Check sheet for the modelled part. Datum: model origin and axes. Units: mm. A direction names the side the tool comes from. Give positions to 0.01 mm unless a question says otherwise; leave off trailing zeros. Order: outer loops, then holes, each group sorted by start corner. A loop starts at its lowest first (then second) coordinate and runs counter-clockwise, first axis right, second up. Notation, with made-up numbers: (84.5, 45.25) - (130.5, 45.25) arc R13 cw to (130.5, 69.25) - close; hole circle Ø9 at (-12, -22.75). An arc over 180 degrees is marked (long way). Answer in a Markdown table with one row per item.
from build123d import *

# Parameters (mm, degrees)
BOSS_EXTRUDE1_DEPTH = 80
SKETCH2_R           = 9
CUT_EXTRUDE1_DEPTH  = 80
SKETCH5_R           = 35
CUT_EXTRUDE2_DEPTH  = 40


with BuildPart() as part:
    # Sketch1 → Boss-Extrude1 (new body)
    with BuildSketch(Plane.XY):
        with BuildLine():
            Line((-99.017681729, 6.463654224), (-99.017681729, -13.536345776))
            Line((-99.017681729, -13.536345776), (40.982318271, -13.536345776))
            Line((40.982318271, -13.536345776), (40.982318271, 6.463654224))
            Line((40.982318271, 6.463654224), (16.110019646, 6.463654224))
            Line((16.110019646, 6.463654224), (16.110019646, 86.463654224))
            Line((16.110019646, 86.463654224), (-3.889980354, 86.463654224))
            ThreePointArc((-3.889980354, 86.463654224), (-33.889980354, 56.463654224), (-63.889980354, 86.463654224))
            Line((-63.889980354, 86.463654224), (-83.889980354, 86.463654224))
            Line((-83.889980354, 86.463654224), (-83.889980354, 6.463654224))
            Line((-83.889980354, 6.463654224), (-99.017681729, 6.463654224))
        make_face()
    extrude(amount=-BOSS_EXTRUDE1_DEPTH)

    # Sketch2 → Cut-Extrude1 (cut)
    with BuildSketch(Plane(origin=(0, 86.463654224, 0), x_dir=(1, 0, 0), z_dir=(0, 1, 0))):
        with Locations((16.110019646, 40)):
            Circle(SKETCH2_R)
        with Locations((-83.889980354, 40)):
            Circle(SKETCH2_R)
    extrude(amount=-CUT_EXTRUDE1_DEPTH, mode=Mode.SUBTRACT)


with BuildPart() as part_1:
    # Body-Move/Copy1: moved
    add(part.part.moved(Location((0, 0, 20))))

    # Sketch5 → Cut-Extrude2 (cut)
    with BuildSketch(Plane.XY):
        with Locations((-33.889980354, 86.463654224)):
            Circle(SKETCH5_R)
    extrude(amount=-CUT_EXTRUDE2_DEPTH, mode=Mode.SUBTRACT)


solid = part_1.part
(1) Cross-section at A-A, the plane z = -36.5. Record the cut outline in (x, y).
Geometry says:
| item | result |
|---|---|
| outline | (-99.02, -13.54) - (40.98, -13.54) - (40.98, 6.46) - (16.11, 6.46) - (16.11, 86.46) - (1.11, 86.46) arc R35 cw to (-68.89, 86.46) - (-83.89, 86.46) - (-83.89, 6.46) - (-99.02, 6.46) - close |
(2) Gauge pin test, flat ends, axial feed: P1, Ø6, axis at y = 13, z = -6.5, coming from the +X side; P2, Ø6, axis at y = 17.5, z = -29.5, coming from the -X side; P3, Ø6, axis at x = -11, z = -43, coming from the +Y side. Record the tip position at first contact, or that the pin passes through.
Geometry says:
| item | result |
|---|---|
| P1 | x = 16.11 |
| P2 | x = -83.89 |
| P3 | y = 71.31 |
(3) Thickness scan on L1, parallel to Z at x = -6.5, y = 74; L2, parallel to Y at x = -89, z = -39; L3, parallel to X at y = 33.5, z = 5. Record the ranges inside material, lowest first.
Geometry says:
| item | result |
|---|---|
| L1 | -60 to -40, 0 to 20 |
| L2 | -13.54 to 6.46 |
| L3 | -83.89 to 16.11 |
(4) Access from +Z, -Z, +X, -X, +Y, -Y to the whole of each face (thin tool, end or side, straight path). Record for faces 4 (the flat face through (16.11, 46, -44)), 5 (the flat face through (-30, 26, -60)), 6 (the flat face through (-34, 56, 0)), 7 (the flat face through (40.982, -4, -19)), 8 (the flat face through (-83.89, 47, 5)).
Geometry says:
| item | result |
|---|---|
| face 4 | +Z, -Z, +X, +Y |
| face 5 | -Z, +X, -X, +Y, -Y |
| face 6 | +Y |
| face 7 | +Z, -Z, +X, +Y, -Y |
| face 8 | +Z, -Z, -X, +Y |
(5) Mould release check, pull along Z, two halves, no side actions. Record for faces 1 (the cylindrical face through (7.112, 47.024, -20.198)), 2 (the flat face through (-30, 26, 20)), 3 (the flat face through (-99.018, -3, -19)): pulls with the +Z half, pulls with the -Z half, needs draft (parallel to the pull), parting line crosses it, or undercut.
Geometry says:
| item | result |
|---|---|
| face 1 | undercut |
| face 2 | pulls with the +Z half |
| face 3 | needs draft |
(6) Cross-section at C-C, the plane x = -31.5. Record the cut outline in (y, z).
Geometry says:
| item | result |
|---|---|
| outline | (-13.54, -60) - (56.56, -60) - (56.56, -40) - (51.55, -40) - (51.55, 0) - (56.56, 0) - (56.56, 20) - (-13.54, 20) - close |
(7) Cross-section at B-B, the plane y = 31.5. Record the cut outline in (x, z).
Geometry says:
| item | result |
|---|---|
| outline | (-83.89, -60) - (16.11, -60) - (16.11, -29) arc R9 cw to (16.11, -11) - (16.11, 20) - (-83.89, 20) - (-83.89, -11) arc R9 cw to (-83.89, -29) - close |
(8) Cross-section at D-D, the plane y = 54.5. Record the cut outline in (x, z).
Geometry says:
| item | result |
|---|---|
| outline | (-83.89, -60) - (16.11, -60) - (16.11, -29) arc R9 cw to (16.11, -11) - (16.11, 20) - (-83.89, 20) - (-83.89, -11) arc R9 cw to (-83.89, -29) - close; hole (-48.15, -40) - (-19.63, -40) - (-19.63, 0) - (-48.15, 0) - close |
